```python
from build123d import *

# Parameters (mm, degrees)
SKETCH_2_W          = 20
SKETCH_2_H          = 40
EXTRUDE_6_DEPTH     = 500
SKETCH_3_R          = 6
CUT_EXTRUDE_1_DEPTH = 502.697119784
SKETCH_5_R          = 3.5
CUT_EXTRUDE_2_DEPTH = 501.799361022


with BuildPart() as part:
    # Эскиз2 → Бобышка-Вытянуть6 (new body)
    with BuildSketch(Plane.XY):
        Rectangle(SKETCH_2_W, SKETCH_2_H)
    extrude(amount=EXTRUDE_6_DEPTH)

    # Эскиз3 → Вырез-Вытянуть1 (cut, through all)
    with BuildSketch(Plane(origin=(0, 20, 0), x_dir=(1, 0, 0), z_dir=(0, 1, 0))):
        with Locations(Location((0, -30, 0), (0, 0, 270))):
            Circle(SKETCH_3_R)
    extrude(amount=-CUT_EXTRUDE_1_DEPTH, mode=Mode.SUBTRACT)

    # Эскиз5 → Вырез-Вытянуть2 (cut, through all)
    with BuildSketch(Plane.ZY.offset(10)):
        with Locations(Location((160, 0, 0), (0, 0, 270))):
            Circle(SKETCH_5_R)
    extrude(amount=-CUT_EXTRUDE_2_DEPTH, mode=Mode.SUBTRACT)


solid = part.part
```
Input: part model. Units: mm. Frame: model coordinates. Give positions to 0.01 mm unless a question says otherwise; leave off trailing zeros. Loops run counter-clockwise (first coordinate to the right, second up) from the corner with the lowest first, then second, coordinate; pieces in that order, holes last.
1) Line query: L1, parallel to X at y = -4, z = 30; L2, parallel to Z at x = 5.25, y = 0; L3, parallel to Z at x = -1, y = 1. Output: solid intervals per line, ascending.
A:
L1: x = -10 to -6, 6 to 10
L2: z = 0 to 27.1, 32.9 to 156.5, 163.5 to 500
L3: z = 0 to 24.08, 35.92 to 156.65, 163.35 to 500
2) Mould query, pull axis Z, two halves, no side actions, for faces 1 (the flat face through (0, 0, 0)), 2 (the flat face through (10, 0, 246)), 3 (the cylindrical face through (0, 0, 24)). Classes: released by +Z, released by -Z, zero draft, split by the parting line, or undercut.
A:
face 1: released by -Z
face 2: zero draft
face 3: undercut
3) Section query B-B on z = 30. Return the cut outline in (x, y).
A:
outline: (-10, -20) - (-6, -20) - (-6, 20) - (-10, 20) - close; (6, -20) - (10, -20) - (10, 20) - (6, 20) - close
4) Section query A-A on x = 0. Return the cut outline in (y, z).
A:
outline: (-20, 0) - (20, 0) - (20, 24) - (-20, 24) - close; (-20, 36) - (20, 36) - (20, 500) - (-20, 500) - close; hole circle Ø7 at (0, 160)
